from build123d import *

# Parameters (mm, degrees)
SKETCH2_W           = 27
SKETCH2_H           = 27
BOSS_EXTRUDE1_DEPTH = 8
SKETCH5_R           = 0.65
CUT_EXTRUDE2_DEPTH  = 8
SKETCH2_6_W         = 27
SKETCH2_6_H         = 27
SKETCH2_6_W_2       = 20
SKETCH2_6_H_2       = 20
BOSS_EXTRUDE2_DEPTH = 43


with BuildPart() as part:
    # Sketch2 → Boss-Extrude1 (new body)
    with BuildSketch(Plane.XY.offset(43)):
        Rectangle(SKETCH2_W, SKETCH2_H)
    extrude(amount=BOSS_EXTRUDE1_DEPTH)

    # Sketch5 → Cut-Extrude2 (cut)
    with BuildSketch(Plane.XY.offset(43)):
        with Locations((-8.23, 8.23)):
            Circle(SKETCH5_R)
        with Locations((-5.88, 8.23)):
            Circle(SKETCH5_R)
        with Locations((-3.53, 8.23)):
            Circle(SKETCH5_R)
        with Locations((-1.18, 8.23)):
            Circle(SKETCH5_R)
        with Locations((1.17, 8.23)):
            Circle(SKETCH5_R)
        with Locations((3.52, 8.23)):
            Circle(SKETCH5_R)
        with Locations((5.87, 8.23)):
            Circle(SKETCH5_R)
        with Locations((8.22, 8.23)):
            Circle(SKETCH5_R)
        with Locations((-5.88, 5.88)):
            Circle(SKETCH5_R)
        with Locations((-3.53, 5.88)):
            Circle(SKETCH5_R)
        with Locations((-1.18, 5.88)):
            Circle(SKETCH5_R)
        with Locations((1.17, 5.88)):
            Circle(SKETCH5_R)
        with Locations((3.52, 5.88)):
            Circle(SKETCH5_R)
        with Locations((5.87, 5.88)):
            Circle(SKETCH5_R)
        with Locations((8.22, 5.88)):
            Circle(SKETCH5_R)
        with Locations((-5.88, 3.53)):
            Circle(SKETCH5_R)
        with Locations((-3.53, 3.53)):
            Circle(SKETCH5_R)
        with Locations((-1.18, 3.53)):
            Circle(SKETCH5_R)
        with Locations((1.17, 3.53)):
            Circle(SKETCH5_R)
        with Locations((3.52, 3.53)):
            Circle(SKETCH5_R)
        with Locations((5.87, 3.53)):
            Circle(SKETCH5_R)
        with Locations((8.22, 3.53)):
            Circle(SKETCH5_R)
        with Locations((-5.88, 1.18)):
            Circle(SKETCH5_R)
        with Locations((-3.53, 1.18)):
            Circle(SKETCH5_R)
        with Locations((-1.18, 1.18)):
            Circle(SKETCH5_R)
        with Locations((1.17, 1.18)):
            Circle(SKETCH5_R)
        with Locations((3.52, 1.18)):
            Circle(SKETCH5_R)
        with Locations((5.87, 1.18)):
            Circle(SKETCH5_R)
        with Locations((8.22, 1.18)):
            Circle(SKETCH5_R)
        with Locations((-5.88, -1.17)):
            Circle(SKETCH5_R)
        with Locations((-3.53, -1.17)):
            Circle(SKETCH5_R)
        with Locations((-1.18, -1.17)):
            Circle(SKETCH5_R)
        with Locations((1.17, -1.17)):
            Circle(SKETCH5_R)
        with Locations((3.52, -1.17)):
            Circle(SKETCH5_R)
        with Locations((5.87, -1.17)):
            Circle(SKETCH5_R)
        with Locations((8.22, -1.17)):
            Circle(SKETCH5_R)
        with Locations((-5.88, -3.52)):
            Circle(SKETCH5_R)
        with Locations((-3.53, -3.52)):
            Circle(SKETCH5_R)
        with Locations((-1.18, -3.52)):
            Circle(SKETCH5_R)
        with Locations((1.17, -3.52)):
            Circle(SKETCH5_R)
        with Locations((3.52, -3.52)):
            Circle(SKETCH5_R)
        with Locations((5.87, -3.52)):
            Circle(SKETCH5_R)
        with Locations((8.22, -3.52)):
            Circle(SKETCH5_R)
        with Locations((-5.88, -5.87)):
            Circle(SKETCH5_R)
        with Locations((-3.53, -5.87)):
            Circle(SKETCH5_R)
        with Locations((-1.18, -5.87)):
            Circle(SKETCH5_R)
        with Locations((1.17, -5.87)):
            Circle(SKETCH5_R)
        with Locations((3.52, -5.87)):
            Circle(SKETCH5_R)
        with Locations((5.87, -5.87)):
            Circle(SKETCH5_R)
        with Locations((8.22, -5.87)):
            Circle(SKETCH5_R)
        with Locations((-5.88, -8.22)):
            Circle(SKETCH5_R)
        with Locations((-3.53, -8.22)):
            Circle(SKETCH5_R)
        with Locations((-1.18, -8.22)):
            Circle(SKETCH5_R)
        with Locations((1.17, -8.22)):
            Circle(SKETCH5_R)
        with Locations((3.52, -8.22)):
            Circle(SKETCH5_R)
        with Locations((5.87, -8.22)):
            Circle(SKETCH5_R)
        with Locations((8.22, -8.22)):
            Circle(SKETCH5_R)
        with Locations((-8.23, 5.88)):
            Circle(SKETCH5_R)
        with Locations((-8.23, 3.53)):
            Circle(SKETCH5_R)
        with Locations((-8.23, 1.18)):
            Circle(SKETCH5_R)
        with Locations((-8.23, -1.17)):
            Circle(SKETCH5_R)
        with Locations((-8.23, -3.52)):
            Circle(SKETCH5_R)
        with Locations((-8.23, -5.87)):
            Circle(SKETCH5_R)
        with Locations((-8.23, -8.22)):
            Circle(SKETCH5_R)
    extrude(amount=CUT_EXTRUDE2_DEPTH, mode=Mode.SUBTRACT)

    # Sketch2<6> → Boss-Extrude2 (add)
    with BuildSketch(Plane.XY.offset(43)):
        Rectangle(SKETCH2_6_W, SKETCH2_6_H)
        Rectangle(SKETCH2_6_W_2, SKETCH2_6_H_2, mode=Mode.SUBTRACT)
    extrude(amount=-BOSS_EXTRUDE2_DEPTH)


solid = part.part
Geometry: final body of the model. Coordinates: model frame, mm. Give positions to 0.01 mm unless a question says otherwise; leave off trailing zeros. Order: outer loops, then holes, each group sorted by start corner. A loop starts at its lowest first (then second) coordinate and runs counter-clockwise, first axis right, second up. Notation, with made-up numbers: (59, 35) - (97, 35) arc R18 cw to (97, 63) - close; hole circle Ø3 at (6.5, -17.75). An arc over 180 degrees is marked (long way). Use CSV: the item, a comma, the result in double quotes.
1. Contact query for flat-ended pins moving along their axis: pin 1 (1.5 mm diameter, centred on x = 8.22, y = -5.87, fed in from -Z); pin 2 (1.2 mm diameter, centred on x = 3.52, y = 5.88, fed in from -Z). Output: stop coordinate, or through.
Answers below:
pin 1,"z = 43"
pin 2,"through"
2. Section query A-A (z = 14). Output: boundary loops of the cut face in (x, y).
Answers below:
outline,"(-13.5, -13.5) - (13.5, -13.5) - (13.5, 13.5) - (-13.5, 13.5) - close; hole (-10, -10) - (10, -10) - (10, 10) - (-10, 10) - close"
3. Material intervals for line 1 along X through (y, z) = (2.75, 14); line 2 along Z through (x, y) = (-4.5, -7.25), sorted ascending. Write a range as from..to.
Answers below:
line 1,"-13.5..-10, 10..13.5"
line 2,"43..51"
4. Mould query, pull axis X, two halves, no side actions, for faces 1 (the face through (0, 13.5, 26)), 2 (the face through (-3.615, 6.524, 46.944)). Classes: +X half, -X half, draft (parallel to the pull), parting line (faces both ways), or undercut.
Answers below:
face 1,"draft"
face 2,"undercut"
5. Section query B-B (y = 5.88). Give the number of separate pieces and of enclosed holes in the cut face, plus the area to 3 significant figures.
Answers below:
separate pieces,"9"
enclosed holes,"0"
area,"434 mm2"
